Read the model definition and answer for the solid it produces. Units are mm, in the model's axes. Face numbers are marked on the shaded views. Round coordinates to 2 decimals unless told otherwise and drop trailing zeros. Order: outer loops, then holes, each group sorted by start corner. A loop starts at its lowest first (then second) coordinate and runs counter-clockwise, first axis right, second up. Notation, with made-up numbers: (21, -21.5) - (75, -21.5) arc R35 cw to (75, 10.5) - close; hole circle Ø2 at (-19.75, -8.5). An arc over 180 degrees is marked (long way). One line per question, with ' | ' between items. Start each with the question number.
1) The part is cut by section A-A, the plane x = -5.5. Give the vertices of the cut face in (y, z).
2) Straight lines are drawn through the part: line 1 (Z direction, x = 0, y = 0.15); line 2 (X direction, y = 0.05, z = 0); line 3 (X direction, y = 0.6, z = 7). For each, find the intervals that lie inside material, in ascending order. Write a range as from..to.
3) The mould has two halves that part along Z. Classify the marked faces 1 and 2: pulls with the +Z half, pulls with the -Z half, needs draft (parallel to the pull), parting line crosses it, or undercut.
4) Flat-ended cylindrical pins translate along their axes: pin 1 (14.5 mm diameter, centred on x = 0, z = 0, fed in from +Y); pin 2 (1.5 mm diameter, centred on x = -5.5, y = -1, fed in from -Z). Find the tip coordinate at first contact, or state that the pin passes through.
5) The part is cut by section D-D, the plane x = 3.5. Give the vertices of the cut face in (y, z).
6) The part is cut by section B-B, the plane z = 0. Give the vertices of the cut face in (x, y), plus the area to 3 significant figures.
7) The part is cut by section C-C, the plane z = 10. Give the vertices of the cut face in (x, y), plus the area to 3 significant figures.
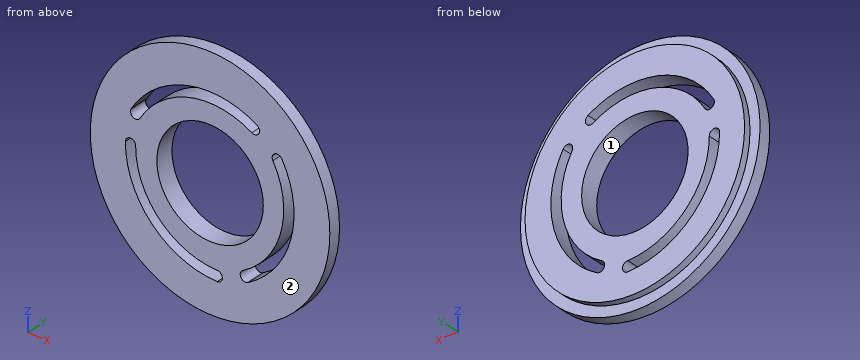
from build123d import *

# Parameters (mm, degrees)
SKETCH1_R           = 18
BOSS_EXTRUDE2_DEPTH = 1.8
SKETCH2_R           = 16.5
BOSS_EXTRUDE3_DEPTH = 1
SKETCH3_R           = 8
CUT_EXTRUDE1_DEPTH  = 5
CUT_EXTRUDE2_DEPTH  = 5


with BuildPart() as part:
    # Sketch1 → Boss-Extrude2 (new body)
    with BuildSketch(Plane(origin=(0, 0, 0), x_dir=(1, 0, 0), z_dir=(0, 1, 0))):
        Circle(SKETCH1_R)
    extrude(amount=-BOSS_EXTRUDE2_DEPTH)

    # Sketch2 → Boss-Extrude3 (add)
    with BuildSketch(Plane(origin=(0, 0, 0), x_dir=(1, 0, 0), z_dir=(0, 1, 0))):
        Circle(SKETCH2_R)
    extrude(amount=BOSS_EXTRUDE3_DEPTH)

    # Sketch3 → Cut-Extrude1 (cut)
    with BuildSketch(Plane(origin=(0, 1, 0), x_dir=(1, 0, 0), z_dir=(0, 1, 0))):
        Circle(SKETCH3_R)
    extrude(amount=-CUT_EXTRUDE1_DEPTH, mode=Mode.SUBTRACT)

    # Sketch5 → Cut-Extrude2 (cut)
    with BuildSketch(Plane(origin=(0, 1, 0), x_dir=(1, 0, 0), z_dir=(0, 1, 0))):
        with BuildLine():
            ThreePointArc((1.075948411, 13.068091917), (-8.698835605, 9.002564361), (-12.735889562, -0.784013805))
            ThreePointArc((-12.735889562, -0.784013805), (-11.960287094, -1.557361616), (-11.186939283, -0.781759147))
            ThreePointArc((-11.186939283, -0.781759147), (-7.601968074, 7.908885399), (1.078203069, 11.519141638))
            ThreePointArc((1.078203069, 11.519141638), (1.85155088, 12.294744107), (1.075948411, 13.068091917))
        make_face()
        with BuildLine():
            ThreePointArc((10.779325374, -7.465844616), (12.145867238, 3.032130437), (5.688968909, 11.421610803))
            ThreePointArc((5.688968909, 11.421610803), (4.631428825, 11.136593267), (4.916446361, 10.079053183))
            ThreePointArc((4.916446361, 10.079053183), (10.650279708, 2.629054772), (9.436767754, -6.693322067))
            ThreePointArc((9.436767754, -6.693322067), (9.72178529, -7.750862152), (10.779325374, -7.465844616))
        make_face()
        with BuildLine():
            ThreePointArc((-11.855273785, -5.602247302), (-3.447031633, -12.034694797), (7.046920653, -10.637596998))
            ThreePointArc((7.046920653, -10.637596998), (7.328858269, -9.579231652), (6.270492922, -9.297294036))
            ThreePointArc((6.270492922, -9.297294036), (-3.048311634, -10.537940171), (-10.514970823, -4.825819571))
            ThreePointArc((-10.514970823, -4.825819571), (-11.573336169, -4.543881955), (-11.855273785, -5.602247302))
        make_face()
    extrude(amount=-CUT_EXTRUDE2_DEPTH, mode=Mode.SUBTRACT)


solid = part.part
Values:
1) outline: (-1.8, -17.14) - (0, -17.14) - (0, -15.56) - (1, -15.56) - (1, -11.39) - (-1.8, -11.39) - close; (-1.8, -9.6) - (1, -9.6) - (1, -5.81) - (-1.8, -5.81) - close; (-1.8, 5.81) - (1, 5.81) - (1, 9.59) - (-1.8, 9.59) - close; (-1.8, 11.31) - (1, 11.31) - (1, 15.56) - (0, 15.56) - (0, 17.14) - (-1.8, 17.14) - close
2) line 1: z = -16.5..-13.02, -11.47..-8, 8..10.95, 12.5..16.5 | line 2: x = -16.5..-12.71, -11.16..-8, 8..11.06, 12.61..16.5 | line 3: x = -14.94..-10.93, -8.91..-3.87, 3.87..9.34, 11.04..14.94
3) face 1: undercut | face 2: needs draft
4) pin 1: passes through | pin 2: stops at z = -17.36
5) outline: (-1.8, -17.66) - (0, -17.66) - (0, -16.12) - (1, -16.12) - (1, -7.19) - (-1.8, -7.19) - close; (-1.8, 7.19) - (1, 7.19) - (1, 10.48) - (-1.8, 10.48) - close; (-1.8, 12.08) - (1, 12.08) - (1, 16.12) - (0, 16.12) - (0, 17.66) - (-1.8, 17.66) - close
6) outline: (-18, -1.8) - (-12.71, -1.8) - (-12.71, 1) - (-16.5, 1) - (-16.5, 0) - (-18, 0) - close; (-11.16, -1.8) - (-8, -1.8) - (-8, 1) - (-11.16, 1) - close; (8, -1.8) - (11.06, -1.8) - (11.06, 1) - (8, 1) - close; (12.61, -1.8) - (18, -1.8) - (18, 0) - (16.5, 0) - (16.5, 1) - (12.61, 1) - close | area: 44.3 mm^2
7) outline: (-14.97, -1.8) - (-7.82, -1.8) - (-7.82, 1) - (-13.12, 1) - (-13.12, 0) - (-14.97, 0) - close; (-4.63, -1.8) - (4.85, -1.8) - (4.85, 1) - (-4.63, 1) - close; (7.43, -1.8) - (14.97, -1.8) - (14.97, 0) - (13.12, 0) - (13.12, 1) - (7.43, 1) - close | area: 64.0 mm^2
